Source: CAD feature listing. Evaluate the final solid. Frame: model axes, mm. A direction names the side the tool comes from. Give positions to 0.01 mm unless a question says otherwise; leave off trailing zeros. Loops run counter-clockwise (first coordinate to the right, second up) from the corner with the lowest first, then second, coordinate; pieces in that order, holes last. Notation, with made-up numbers: M -24,86 L 8,86 A12 cw 8,101 Z; hole C 38,46.25 d4. An arc over 180 degrees is marked long. Put each result on its own line as item: value. Start each with the question number.
```python
from build123d import *

# Parameters (mm, degrees)
F0_W     = 121.5
F0_H     = 74.1
F1_DEPTH = 30
F2_T     = -2.5
F5_DEPTH = 79.2


with BuildPart() as f1:
    # F0 (on Top) → F1 (new body)
    with BuildSketch(Plane.XY):
        Rectangle(F0_W, F0_H)
    extrude(amount=F1_DEPTH)

    # F2
    f2_openings = [f1.faces().sort_by_distance(p)[0] for p in [
        (0, 0, 30),
    ]]
    offset(amount=F2_T, openings=f2_openings)

    # F3 (on face) → F5 (cut)
    with BuildSketch(Plane(origin=(0, 37.05, 0), x_dir=(-1, 0, 0), z_dir=(0, 1, 0))):
        Polygon((-60.75, 19.370127), (60.75, 30), (-60.75, 30), align=None)
    extrude(amount=-F5_DEPTH, mode=Mode.SUBTRACT)


solid = f1.part
```
1. Ray query, line 1 (X direction, y = 8, z = 13); line 2 (Y direction, x = -49.5, z = 20.5); line 3 (Z direction, x = 43, y = 20.5). Return the intervals inside material, ascending.
2. Pull-direction query (Y, two-part tool) for faces 1 (the face through (58.25, 0, 11)), 2 (the face through (-1, 37.05, 11)), 3 (the face through (-1, 0, 2.5)), 4 (the face through (-1, 1, 0)); classes: released by +Y, released by -Y, zero draft, split by the parting line, or undercut.
3. Set-up query: faces 5 (the face through (-1, 34.55, 13)), 6 (the face through (60.75, -1, 10)). Return all of +Z, -Z, +X, -X, +Y, -Y with unobstructed straight access to the full face (end or side cutting, diameter ignored); none if empty.
4. Contact query for flat-ended pins moving along their axis: pin 1 (13.5 mm diameter, centred on y = 1, z = 22.5, fed in from +X); pin 2 (3 mm diameter, centred on x = 35.5, y = -13, fed in from +Z). Output: stop coordinate, or through.
5. Section C-C, the plane x = -14.5. Output: boundary loops of the cut face in (y, z).
6. Section A-A, the plane z = 13. Output: boundary loops of the cut face in (x, y), plus the area to 3 significant figures.
7. Section B-B, the plane y = 13. Output: boundary loops of the cut face in (x, z), plus the area to 3 significant figures.
Results found:
1. line 1: -60.75 to -58.25, 58.25 to 60.75
1. line 2: -37.05 to -34.55, 34.55 to 37.05
1. line 3: 0 to 2.5
2. face 1: undercut
2. face 2: released by +Y
2. face 3: undercut
2. face 4: zero draft
3. face 5: +Z
3. face 6: +Z, -Z, +X, +Y, -Y
4. pin 1: x = 60.75
4. pin 2: z = 2.5
5. outline: M -37.05,0 L 37.05,0 L 37.05,25.95 L 34.55,25.95 L 34.55,2.5 L -34.55,2.5 L -34.55,25.95 L -37.05,25.95 Z
6. outline: M -60.75,-37.05 L 60.75,-37.05 L 60.75,37.05 L -60.75,37.05 Z; hole M -58.25,-34.55 L 58.25,-34.55 L 58.25,34.55 L -58.25,34.55 Z
6. area: 953 mm²
7. outline: M -60.75,0 L 60.75,0 L 60.75,19.37 L 58.25,19.59 L 58.25,2.5 L -58.25,2.5 L -58.25,29.78 L -60.75,30 Z
7. area: 415 mm²
